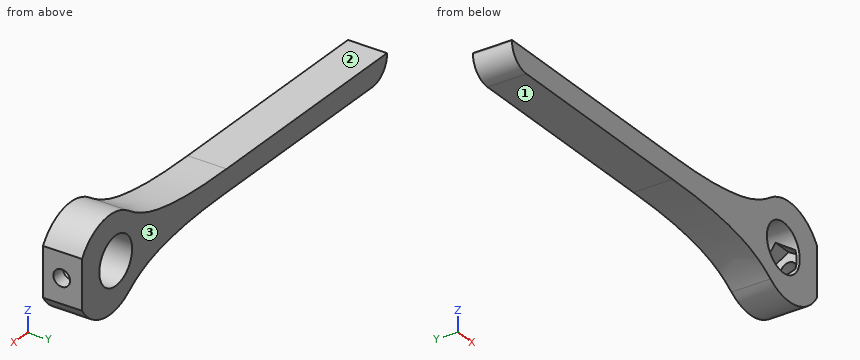
from build123d import *

# Parameters (mm, degrees)
SKETCH1_R               = 4.3
BOSS_EXTRUDE1_DEPTH     = 7
CUT_EXTRUDE1_REACH      = 82.754
CUT_EXTRUDE1_END_RADIUS = 4.3
SKETCH2_R               = 1.496285127
CUT_EXTRUDE3_START      = -7
CUT_EXTRUDE3_DEPTH      = 4.5


with BuildPart() as part:
    # Sketch1 → Boss-Extrude1 (new body)
    with BuildSketch(Plane(origin=(0, 0, 0), x_dir=(1, 0, 0), z_dir=(0, 1, 0))):
        with BuildLine():
            Line((-71.170433536, -2), (-29.082351877, -2))
            add(Edge.make_bspline(
                [(-29.082351877, -2), (-23.609649847, -2), (-15.245438708, -2.238584536), (-6.627824546, -4.603953255), (-3.36619416, -6.925224681)],
                knots=[0, 0, 0, 0, 0.607849165, 1, 1, 1, 1], degree=3))
            ThreePointArc((-3.36619416, -6.925224681), (3.28001342, -8.324655054), (8.829566464, -4.408925038))
            Line((8.829566464, -4.408925038), (8.829566464, 4.408925038))
            ThreePointArc((8.829566464, 4.408925038), (3.28001342, 8.324655054), (-3.36619416, 6.925224681))
            add(Edge.make_bspline(
                [(-29.082351877, 2), (-23.609649847, 2), (-15.245438708, 2.238584536), (-6.627824546, 4.603953255), (-3.36619416, 6.925224681)],
                knots=[0, 0, 0, 0, 0.607849165, 1, 1, 1, 1], degree=3))
            Line((-29.082351877, 2), (-67.370433536, 2))
            ThreePointArc((-67.370433536, 2), (-70.057439304, 0.887005769), (-71.170433536, -1.8))
            Line((-71.170433536, -1.8), (-71.170433536, -2))
        make_face()
        with Locations(Location((0, 0, 0), (0, 0, 270))):
            Circle(SKETCH1_R, mode=Mode.SUBTRACT)
    extrude(amount=BOSS_EXTRUDE1_DEPTH)

    # Cut-Extrude1: up to this cylinder (the profile starts outside it)
    cut_extrude1_end = Plane(origin=(0, 3.358684, 0), z_dir=(0, -1, 0)) * Cylinder(CUT_EXTRUDE1_END_RADIUS, 175.108, mode=Mode.PRIVATE)
    # Sketch2 → Cut-Extrude1 (cut, up to the surface)
    with BuildSketch(Plane(origin=(8.829566464, 0, 0), x_dir=(0, 0, -1), z_dir=(1, 0, 0)), mode=Mode.PRIVATE) as cut_extrude1_sk1:
        with Locations((0, 3.358684182)):
            Circle(SKETCH2_R)
    cut_extrude1_tool1 = extrude(cut_extrude1_sk1.sketch, amount=-CUT_EXTRUDE1_REACH, mode=Mode.PRIVATE) - cut_extrude1_end
    add(cut_extrude1_tool1.solids().sort_by_distance((8.829566, 3.358684, 0))[0], mode=Mode.SUBTRACT)

    # Sketch3 → Cut-Extrude3 (cut)
    with BuildSketch(Plane(origin=(8.829566464, 0, 0), x_dir=(0, 0, -1), z_dir=(1, 0, 0)).offset(CUT_EXTRUDE3_START)):
        Polygon((-1.615510912, 0.560537202), (1.615510912, 0.560537202), (3.231021825, 3.358684182), (1.615510912, 6.156831163), (-1.615510912, 6.156831163), (-3.231021825, 3.358684182), align=None)
    extrude(amount=CUT_EXTRUDE3_DEPTH, mode=Mode.SUBTRACT)


solid = part.part
Build history of the part. All positions in model axes, mm. Face numbers are marked on the shaded views. A direction names the side the tool comes from. Coordinates: 2 decimals unless noted, no trailing zeros. Order: outer loops, then holes, each group sorted by start corner. A loop starts at its lowest first (then second) coordinate and runs counter-clockwise, first axis right, second up. Notation, with made-up numbers: (8, -26.75) - (28, -26.75) arc R9 cw to (28, -10.75) - close; hole circle Ø9 at (18, -5). An arc over 180 degrees is marked (long way). Write item = value, one per line. Start each with the question number.
1) Wall check: line 1 along Y through (x, z) = (6.9, 0); line 2 along Z through (x, y) = (-37, 4.5); line 3 along Z through (x, y) = (-1.5, 6.5). Give the ranges that are in metal, low to high. Write a range as from..to.
2) Saw through at C-C on x = -46. Write the cut outline in (y, z), then the cut area to 3 significant figures.
3) Saw through at A-A on x = 0. Write the cut outline in (y, z), then the cut area to 3 significant figures.
4) Flat gauge pins, fed straight in: pin 1 Ø6 at (x, z) = (-55, 6.5) entering from +Y; pin 2 Ø1 at (x, y) = (-34, 3.5) entering from -Z. Where does each tip first touch, or does it go through?
5) 3-axis set-ups, long thin cutter, end or side, ignore diameter. For the marked faces 1, 2 and 3: which of +Z, -Z, +X, -X, +Y, -Y reach the whole face in a straight line?
6) Saw through at B-B on z = 0. Write the cut outline in (x, y).
From the geometry:
q1.line_1 = 0..1.86, 4.85..7
q1.line_2 = -2..2
q1.line_3 = -7.93..-4.03, 4.03..7.93
q2.outline = (0, -2) - (7, -2) - (7, 2) - (0, 2) - close
q2.area = 28.0 mm^2
q3.outline = (0, -8.36) - (7, -8.36) - (7, -4.3) - (0, -4.3) - close; (0, 4.3) - (7, 4.3) - (7, 8.36) - (0, 8.36) - close
q3.area = 56.8 mm^2
q4.pin_1 = through
q4.pin_2 = -2
q5.face_1 = -Z, -X, +Y, -Y
q5.face_2 = +Z, -X, +Y, -Y
q5.face_3 = +Z, -Z, +X, -X, +Y
q6.outline = (-70.72, 0) - (-4.3, 0) - (-4.3, 7) - (-70.72, 7) - close; (4.3, 0) - (8.83, 0) - (8.83, 1.86) - (6.33, 1.86) - (6.33, 0.56) - (4.3, 0.56) - close; (4.3, 6.16) - (6.33, 6.16) - (6.33, 4.85) - (8.83, 4.85) - (8.83, 7) - (4.3, 7) - close
